from build123d import *

# Parameters (mm, degrees)
SKETCH1_R           = 50.8
BOSS_EXTRUDE1_DEPTH = 8.89
SKETCH2_W           = 29
SKETCH2_H           = 3
CUT_EXTRUDE2_DEPTH  = 127


with BuildPart() as part:
    # Sketch1 → Boss-Extrude1 (new body)
    with BuildSketch(Plane(origin=(0, 0, 0), x_dir=(1, 0, 0), z_dir=(0, 1, 0))):
        with Locations(Location((0, 0, 0), (0, 0, 90))):
            Circle(SKETCH1_R)
        with BuildLine():
            Line((-29.416294804, 35), (29.416294804, 35))
            ThreePointArc((29.416294804, 35), (0, -45.72), (-29.416294804, 35))
        make_face(mode=Mode.SUBTRACT)
    extrude(amount=BOSS_EXTRUDE1_DEPTH)

    # Sketch2 → Cut-Extrude2 (cut)
    with BuildSketch(Plane(origin=(0, 8.89, 0), x_dir=(1, 0, 0), z_dir=(0, 1, 0))):
        with Locations((0, 39.8)):
            Rectangle(SKETCH2_W, SKETCH2_H)
    extrude(amount=-CUT_EXTRUDE2_DEPTH, mode=Mode.SUBTRACT)


solid = part.part
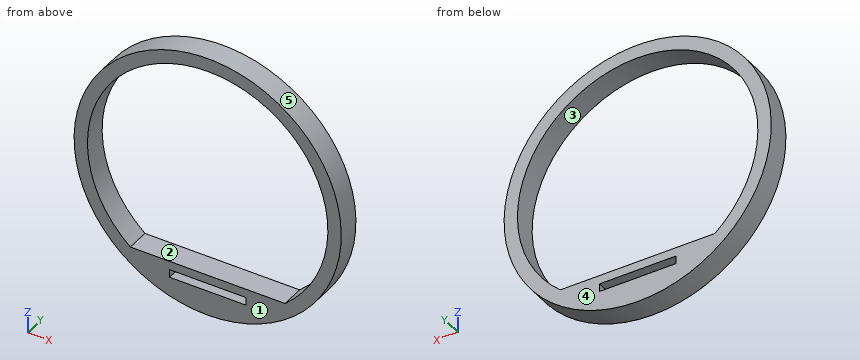
Could you check a few things on this model? Use its own coordinates, in mm. Face numbers are marked on the shaded views. A direction names the side the tool comes from. Round coordinates to 2 decimals unless told otherwise and drop trailing zeros. Order: outer loops, then holes, each group sorted by start corner. A loop starts at its lowest first (then second) coordinate and runs counter-clockwise, first axis right, second up.
Q1. I'm going to push flat-ended pins straight in: P1, Ø4, axis at y = 4, z = -5.5, coming from the -X side; P2, Ø1, axis at y = 5.5, z = 31, coming from the +X side (3 decimals); P3, Ø3.5, axis at y = 6, z = -40.5, coming from the +X side. Where does each tip first touch, or does it pass through?
Geometry says:
P1: stops at x = -50.68
P2: stops at x = 40.625
P3: stops at x = 32.85
Q2. Please list where these lines run through material, in increasing order: probe 1 along Z at (x, y) = (-8, 2); probe 2 along Z at (x, y) = (-6.5, 5); probe 3 along X at (y, z) = (2.5, 0).
Geometry says:
probe 1: z = -50.17 to -41.3, -38.3 to -35, 45.01 to 50.17
probe 2: z = -50.38 to -41.3, -38.3 to -35, 45.26 to 50.38
probe 3: x = -50.8 to -45.72, 45.72 to 50.8
Q3. Imagine slicing it at B-B, the plane y = 2.5. List the corners of the cut face in (x, z) for me, then the cut area to 3 significant figures.
Geometry says:
outline: circle Ø101.6 at (0, 0); hole (-29.42, -35) - (29.42, -35) arc R45.72 ccw (long way) to start; hole (-14.5, -41.3) - (14.5, -41.3) - (14.5, -38.3) - (-14.5, -38.3) - close
area: 1,880 mm2
Q4. Imagine slicing it at C-C, the plane z = 0. List the corners of the cut face in (x, y) for me.
Geometry says:
outline: (-50.8, 0) - (-45.72, 0) - (-45.72, 8.89) - (-50.8, 8.89) - close; (45.72, 0) - (50.8, 0) - (50.8, 8.89) - (45.72, 8.89) - close
Q5. Imagine slicing it at D-D, the plane x = 17.5. List the corners of the cut face in (y, z) for me, then the cut area to 3 significant figures.
Geometry says:
outline: (0, -47.69) - (8.89, -47.69) - (8.89, -35) - (0, -35) - close; (0, 42.24) - (8.89, 42.24) - (8.89, 47.69) - (0, 47.69) - close
area: 161 mm2
Q6. Which directions (+Z, -Z, +X, -X, +Y, -Y) give clear straight access to the entire face, cutting with the end or side of a thin tool? Please do the marked faces 1 and 2.
Geometry says:
face 1: +Z, -Z, +X, -X, -Y
face 2: +Y, -Y
Q7. Thinking about a two-plate mould opening in Z: for the marked faces 3, 4 and 5, which applies, released by +Z, released by -Z, zero draft, split by the parting line, or undercut?
Geometry says:
face 3: undercut
face 4: zero draft
face 5: split by the parting line
Q8. Imagine slicing it at A-A, the plane x = 0. List the corners of the cut face in (y, z) for me, then the cut area to 3 significant figures.
Geometry says:
outline: (0, -50.8) - (8.89, -50.8) - (8.89, -41.3) - (0, -41.3) - close; (0, -38.3) - (8.89, -38.3) - (8.89, -35) - (0, -35) - close; (0, 45.72) - (8.89, 45.72) - (8.89, 50.8) - (0, 50.8) - close
area: 159 mm2
